Read the model definition and answer for the solid it produces. Units are mm, in the model's axes. A direction names the side the tool comes from. Coordinates: 2 decimals unless noted, no trailing zeros. Order: outer loops, then holes, each group sorted by start corner. A loop starts at its lowest first (then second) coordinate and runs counter-clockwise, first axis right, second up. Notation, with made-up numbers: (1, 9.5) - (7, 9.5) arc R31 ccw to (7, 41.5) - close; hole circle Ø4 at (27, 83.25). An arc over 180 degrees is marked (long way). Answer as a JSON object with one key per item and string values. Group by question number.
from build123d import *

# Parameters (mm, degrees)
F0_W      = 20
F0_H      = 20
F1_DEPTH  = 3.6
F2_W      = 6.6
F2_H      = 4
F3_DEPTH  = 25
F5_ANGLE  = 90
F8_DEPTH  = 3.6
F10_DEPTH = 3.6


with BuildPart() as f1:
    # F0 (on Top) → F1 (new body)
    with BuildSketch(Plane.XY):
        with Locations((0, 14)):
            Rectangle(F0_W, F0_H)
    extrude(amount=F1_DEPTH)

    # F2 (on face) → F3 (cut)
    with BuildSketch(Plane.XY.offset(3.6)):
        with BuildLine():
            ThreePointArc((3.3, 13.6), (0, 16.9), (-3.3, 13.6))
            Line((-3.3, 13.6), (3.3, 13.6))
        make_face()
        with Locations((0, 11.6)):
            Rectangle(F2_W, F2_H)
        with BuildLine():
            Line((3.3, 9.6), (-3.3, 9.6))
            ThreePointArc((-3.3, 9.6), (0, 6.3), (3.3, 9.6))
        make_face()
    extrude(amount=-F3_DEPTH, mode=Mode.SUBTRACT)


with BuildPart() as f4_1:
    # F4: instance of F1
    add(f1.part.mirror(Plane(origin=(0, 24, 1.8), x_dir=(-1, 0, 0), z_dir=(0, 1, 0))))


with BuildPart() as f4_1_1:
    # F5: moved
    add(f4_1.part.rotate(Axis((0, 24, 3.6), (-1, 0, 0)), F5_ANGLE))


with BuildPart() as f1_1:
    add(f1.part)

    # F6: union F4_1
    add(f4_1_1.part)

    # F7 (on face) → F8 (join)
    with BuildSketch(Plane.YZ.offset(10)):
        Polygon((20.4, 0), (4, 0), (20.4, -16.4), align=None)
    extrude(amount=-F8_DEPTH)

    # F9 (on face) → F10 (join)
    with BuildSketch(Plane(origin=(-10, 0, 0), x_dir=(0, -1, 0), z_dir=(-1, 0, 0))):
        Polygon((-20.4, -16.4), (-4, 0), (-20.4, 0), align=None)
    extrude(amount=-F10_DEPTH)


solid = f1_1.part
1. For a pull along X with two mould halves and no side action, classify faces 1 (the flat face through (0, 22, -16.4)), 2 (the cylindrical face through (0.1, 16.9, 1.8)), 3 (the flat face through (10, 16, -4)) as pulls with the +X half, pulls with the -X half, needs draft (parallel to the pull), parting line crosses it, or undercut.
2. Straight lines are drawn through the part: L1, parallel to X at y = 21.5, z = -8; L2, parallel to Z at x = 5.5, y = 9.25; L3, parallel to Y at x = 4, z = -1.25. For each, find the intervals that lie inside material, in ascending order.
3. A cutting plane is placed at C-C on y = 18.25. Write down the section's boundary in (x, z).
4. For faces 4 (the flat face through (-4, 20.4, -8)), 5 (the cylindrical face through (-0.1, 22.2, -14.1)), 6 (the flat face through (3.3, 12, 2)), determine the directions among +Z, -Z, +X, -X, +Y, -Y from which every point of the face is accessible in a straight line to the end or side of a thin tool.
5. A cutting plane is placed at B-B on z = -8.5. Write down the section's boundary in (x, y), and give its area (3 significant figures).
6. A cutting plane is placed at A-A on x = 0. Write down the section's boundary in (y, z).
7. A cutting plane is placed at D-D on y = 7.5. Write down the section's boundary in (x, z), and give its area (3 significant figures).
8. Given pin 1 (10 mm diameter, centred on x = 6.5, y = 12, fed in from -Z); pin 2 (1.5 mm diameter, centred on x = -4, z = -5, fed in from -Y); pin 3 (3 mm diameter, centred on x = 7, y = 9.5, fed in from -Z), each flat-ended and moving along its own axis, determine where each tip first touches the part or whether it passes through.
Derived:
{
 "1": {"face 1": "needs draft", "face 2": "undercut", "face 3": "pulls with the +X half"},
 "2": {"L1": "x = -10 to -3.3, 3.3 to 10", "L2": "z = 0 to 3.6", "L3": "y = 20.4 to 24"},
 "3": {"outline": "(-10, -14.25) - (-6.4, -14.25) - (-6.4, 0) - (6.4, 0) - (6.4, -14.25) - (10, -14.25) - (10, 3.6) - (-10, 3.6) - close"},
 "4": {"face 4": "-Z, -Y", "face 5": "+Y, -Y", "face 6": "+Z, -Z"},
 "5": {"outline": "(-10, 12.5) - (-6.4, 12.5) - (-6.4, 20.4) - (-3.3, 20.4) - (-3.3, 24) - (-10, 24) - close; (3.3, 20.4) - (6.4, 20.4) - (6.4, 12.5) - (10, 12.5) - (10, 24) - (3.3, 24) - close", "area": "105 mm2"},
 "6": {"outline": "(4, 0) - (6.3, 0) - (6.3, 3.6) - (4, 3.6) - close; (16.9, 0) - (20.4, 0) - (20.4, -3.5) - (24, -3.5) - (24, 3.6) - (16.9, 3.6) - close; (20.4, -16.4) - (24, -16.4) - (24, -14.1) - (20.4, -14.1) - close"},
 "7": {"outline": "(-10, -3.5) - (-6.4, -3.5) - (-6.4, 0) - (-2.55, 0) - (-2.55, 3.6) - (-10, 3.6) - close; (2.55, 0) - (6.4, 0) - (6.4, -3.5) - (10, -3.5) - (10, 3.6) - (2.55, 3.6) - close", "area": "78.9 mm2"},
 "8": {"pin 1": "stops at z = -13", "pin 2": "stops at y = 20.4", "pin 3": "stops at z = -7"}
}
